Check sheet for the modelled part. Datum: model origin and axes. Units: mm. A direction names the side the tool comes from. Give positions to 0.01 mm unless a question says otherwise; leave off trailing zeros. Order: outer loops, then holes, each group sorted by start corner. A loop starts at its lowest first (then second) coordinate and runs counter-clockwise, first axis right, second up.
Autodesk Inventor part; units mm, degrees
ref_plane "YZ Plane" through (0, 0, 0) normal (1, 0, 0) x (0, 1, 0)
ref_plane "XZ Plane" through (0, 0, 0) normal (0, 1, 0) x (-1, 0, 0)
ref_plane "XY Plane" through (0, 0, 0) normal (0, 0, 1) x (1, 0, 0)
sketch "スケッチ1" plane through (0, 0, 0) normal (0, 0, 1) x (1, 0, 0)
  line L0 (0, 0) -> (0, 2.5)
  line L1 (0, 0) -> (0, -2.5)
  arc A0 (0, 2.5) -> (0, -2.5) centre (0, 0) ccw
  dimension "d0" = 2.5
  dimension "d1" = 2.5
  dimension "d2" = 2.5
revolve "回転1" add sketch "スケッチ1" angle 360 about axis through (0, 0, 0) along (0, 1, 0)
sketch "スケッチ2" plane through (0, 0, 0) normal (0, 0, 1) x (1, 0, 0)
  circle A0 centre (0, 0) radius 1.5
  circle A1 centre (0, 0) radius 2.25
  dimension "d4" = 3
  dimension "d5" = 4.5
extrude "押し出し1" add sketch "スケッチ2" along normal mid plane 5
sketch "スケッチ3" plane through (0, 0, 0) normal (0, 0, 1) x (1, 0, 0)
  circle A0 centre (0, 0) radius 1.5
extrude "押し出し2" cut sketch "スケッチ3" along normal mid plane 5
properties part number "タミヤダンパー部品8.1" material "アセタール樹脂、黒"
(1) Cross-section at C-C on z = 2.05. Enter the section's corners in (x, y).
Response values:
outline: circle Ø4.5 at (0, 0); hole circle Ø3 at (0, 0)
(2) Material ranges on L1, parallel to Y at x = 0, z = -0.95; L2, parallel to Y at x = 0.85, z = -1.3; L3, parallel to X at y = -1.35, z = 0.05, recorded low to high.
Response values:
L1: y = -2.31 to -1.5, 1.5 to 2.31
L2: y = -2.08 to -1.24, 1.24 to 2.08
L3: x = -2.1 to -0.65, 0.65 to 2.1
(3) Cross-section at D-D on y = -1.6. Enter the section's corners in (x, z), then the cut area to 3 significant figures.
Response values:
outline: (-1.58, -2.5) - (1.58, -2.5) - (1.58, -1.09) arc R1.92 ccw to (1.58, 1.09) - (1.58, 2.5) - (-1.58, 2.5) - (-1.58, 1.09) arc R1.92 ccw to (-1.58, -1.09) - close
area: 16.8 mm2
(4) Set-up check for faces 4 (the face through (-0.29, 2.23, -1.78)), 5 (the face through (-2, 0, -2.5)): record each of +Z, -Z, +X, -X, +Y, -Y from which the full face is reachable in a straight line by a thin tool's end or side.
Response values:
face 4: -Z
face 5: -Z, +X, -X, +Y, -Y
(5) Release check for a two-part mould opening along Y. For faces 1 (the face through (-0.29, -2.23, 1.78)), 2 (the face through (-1.5, 0.07, 0.04)), 3 (the face through (-2, 0, 2.5)) record: released by +Y, released by -Y, zero draft, split by the parting line, or undercut.
Response values:
face 1: split by the parting line
face 2: undercut
face 3: zero draft
(6) Cross-section at A-A on y = 0. Enter the section's corners in (x, z), then the cut area to 3 significant figures.
Response values:
outline: (-2.25, -2.5) - (-1.5, -2.5) - (-1.5, 2.5) - (-2.25, 2.5) - (-2.25, 1.09) arc R2.5 ccw to (-2.25, -1.09) - close; (1.5, -2.5) - (2.25, -2.5) - (2.25, -1.09) arc R2.5 ccw to (2.25, 1.09) - (2.25, 2.5) - (1.5, 2.5) - close
area: 8.23 mm2
